Geometry: final body of the model. Coordinates: model frame, mm. A direction names the side the tool comes from. Round coordinates to 2 decimals unless told otherwise and drop trailing zeros. Loops run counter-clockwise (first coordinate to the right, second up) from the corner with the lowest first, then second, coordinate; pieces in that order, holes last. Notation, with made-up numbers: (55.25, -10) - (87.25, -10) arc R24 ccw to (87.25, 22) - close; hole circle Ø7 at (56, 44.25). An arc over 180 degrees is marked (long way). Use CSV: the item, a comma, the result in double quotes.
from build123d import *

# Parameters (mm, degrees)
F1_DEPTH = 30
F3_DEPTH = 30
F5_DEPTH = 30


with BuildPart() as f1:
    # F0 (on Front) → F1 (new body)
    with BuildSketch(Plane.XZ):
        Polygon((0, 441), (0, 0), (20, 0), (30, 382.397638), (30, 432.397638), align=None)
    extrude(amount=F1_DEPTH)

    # F2 (on face) → F3 (cut)
    with BuildSketch(Plane(origin=(0, 0, 0), x_dir=(0, -1, 0), z_dir=(-1, 0, 0))):
        Polygon((0, 382.058233), (0, 0), (10, 0), align=None)
    extrude(amount=-F3_DEPTH, mode=Mode.SUBTRACT)

    # F4 (on face) → F5 (cut)
    with BuildSketch(Plane.XZ.offset(30)):
        Polygon((30, 402.397638), (30, 432.397638), (20, 435.265092), (20, 402.397638), align=None)
        Polygon((0, 441), (0, 402.397638), (10, 402.397638), (10, 438.132546), align=None)
    extrude(amount=-F5_DEPTH, mode=Mode.SUBTRACT)


solid = f1.part
Item 1: Section B-B on z = 140. Return the cut outline in (x, y), plus the area to 3 significant figures.
Final values:
outline,"(0, -30) - (23.66, -30) - (23.66, -6.34) - (0, -6.34) - close"
area,"560 mm²"
Item 2: Material intervals for line 1 (Z direction, x = 2.75, y = -11); line 2 (X direction, y = -8.5, z = 60); line 3 (X direction, y = -19, z = 144), sorted ascending.
Final values:
line 1,"z = 0 to 402.4"
line 2,"x = 0 to 21.57"
line 3,"x = 0 to 23.77"
Item 3: Reachability of faces 1 (the flat face through (5, -15, 402.398)), 2 (the flat face through (15, 0, 404)), 3 (the flat face through (25, -15, 402.398)) from +Z, -Z, +X, -X, +Y, -Y: full face, straight path, thin tool, end or side. Return the list, or none.
Final values:
face 1,"+Z, -X, +Y, -Y"
face 2,"+Z, -Z, +X, -X, +Y"
face 3,"+Z, +X, +Y, -Y"
Item 4: Section D-D on z = 92. Return the cut outline in (x, y).
Final values:
outline,"(0, -30) - (22.41, -30) - (22.41, -7.59) - (0, -7.59) - close"
Item 5: Section C-C on x = 15.5. Return the cut outline in (y, z), plus the area to 3 significant figures.
Final values:
outline,"(-30, 0) - (-10, 0) - (0, 382.06) - (0, 436.56) - (-30, 436.56) - close"
area,"11,200 mm²"
Item 6: Section A-A on y = -14.5. Return the cut outline in (x, z).
Final values:
outline,"(0, 0) - (20, 0) - (30, 382.4) - (30, 402.4) - (20, 402.4) - (20, 435.27) - (10, 438.13) - (10, 402.4) - (0, 402.4) - close"
Item 7: Pin query (flat end, axial travel): P1, Ø1, axis at x = 19.5, y = -5, coming from the +Z side; P2, Ø15, axis at y = -7.5, z = 412.5, coming from the +X side; P3, Ø10, axis at x = 21.5, y = -8, coming from the +Z side. Return the tip coordinate at first contact, or that it passes through.
Final values:
P1,"stops at z = 435.55"
P2,"stops at x = 20"
P3,"stops at z = 436.27"
